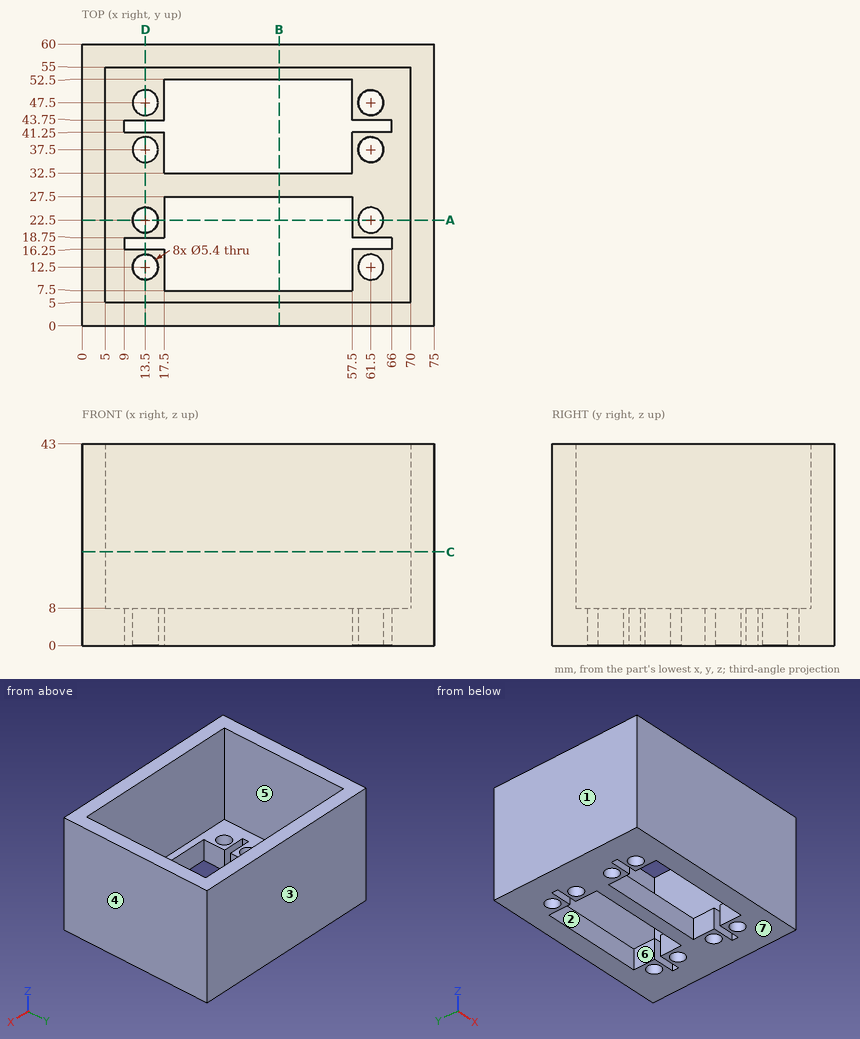
Geometry: see drawing. Coordinates: mm, zero at the bounding-box minimum. A direction names the side the tool comes from. Give positions to 0.01 mm unless a question says otherwise; leave off trailing zeros. Write each loop counter-clockwise with the first axis right and the second up, starting at its lowest first coordinate (ties: lowest second). Pieces come first, ordered by that corner, then holes. Notation, with made-up numbers: (81, -26.5) -> (133, -26.5) arc R15 cw to (133, -14.5) -> close; hole circle Ø5 at (87, 34). An arc over 180 degrees is marked (long way). Use one line per item in the form item = value. Start each with the question number.
1) Draft query along X for the marked faces 1, 2, 3 and 4. Return one class per face: pulls with the +X half, pulls with the -X half, needs draft (parallel to the pull), parting line crosses it, or undercut.
2) Set-up query: the marked faces 5, 6 and 7. Return all of +Z, -Z, +X, -X, +Y, -Y with unobstructed straight access to the full face (end or side cutting, diameter ignored); none if empty.
3) Section query A-A on y = 22.5. Return the cut outline in (x, z), then the cut area to 3 significant figures.
4) Section query D-D on x = 13.5. Count the separate pieces of the cut face and the enclosed holes in it, then the cut area to 3 significant figures.
5) Ray query, probe 1 along Y at (x, z) = (36, 24.5); probe 2 along Y at (x, z) = (57, 7.5); probe 3 along X at (y, z) = (47, 1). Return the intervals inside material, ascending. Write a range as from..to.
6) Section query B-B on x = 42. Return the cut outline in (y, z), then the cut area to 3 significant figures.
7) Section query C-C on z = 20. Return the cut outline in (x, y), then the cut area to 3 significant figures.
8) Pin query (flat end, axial travel): pin 1 (6 mm diameter, centred on x = 61.5, y = 12.5, fed in from +Z). Return the tip coordinate at first contact, or that it passes through.
Outcome:
q1.face_1 = pulls with the -X half
q1.face_2 = undercut
q1.face_3 = needs draft
q1.face_4 = pulls with the +X half
q2.face_5 = +Z
q2.face_6 = +Z, -Z
q2.face_7 = -Z, +X, -X, +Y, -Y
q3.outline = (0, 0) -> (10.8, 0) -> (10.8, 8) -> (5, 8) -> (5, 43) -> (0, 43) -> close; (16.2, 0) -> (17.5, 0) -> (17.5, 8) -> (16.2, 8) -> close; (57.5, 0) -> (58.8, 0) -> (58.8, 8) -> (57.5, 8) -> close; (64.2, 0) -> (75, 0) -> (75, 43) -> (70, 43) -> (70, 8) -> (64.2, 8) -> close
q3.area = 544 mm^2
q4.separate_pieces = 7
q4.enclosed_holes = 0
q4.area = 617 mm^2
q5.probe_1 = 0..5, 55..60
q5.probe_2 = 0..7.5, 27.5..32.5, 52.5..60
q5.probe_3 = 0..10.85, 16.15..17.5, 57.5..58.85, 64.15..75
q6.outline = (0, 0) -> (7.5, 0) -> (7.5, 8) -> (5, 8) -> (5, 43) -> (0, 43) -> close; (27.5, 0) -> (32.5, 0) -> (32.5, 8) -> (27.5, 8) -> close; (52.5, 0) -> (60, 0) -> (60, 43) -> (55, 43) -> (55, 8) -> (52.5, 8) -> close
q6.area = 510 mm^2
q7.outline = (0, 0) -> (75, 0) -> (75, 60) -> (0, 60) -> close; hole (5, 5) -> (70, 5) -> (70, 55) -> (5, 55) -> close
q7.area = 1,250 mm^2
q8.pin_1 = 8
